```python
from build123d import *

# Parameters (mm, degrees)
BOSS_EXTRUDE2_DEPTH = 50
CUT_EXTRUDE2_DEPTH  = 63
SKETCH6_W           = 25
SKETCH6_H           = 16.790562981
BOSS_EXTRUDE4_DEPTH = 16
CUT_EXTRUDE8_DEPTH  = 25
SKETCH11_W          = 19
SKETCH11_H          = 10.094840621
CUT_EXTRUDE9_DEPTH  = 25


with BuildPart() as part:
    # Sketch1 → Boss-Extrude2 (new body)
    with BuildSketch(Plane(origin=(0, 0, 0), x_dir=(1, 0, 0), z_dir=(0, 1, 0))):
        Polygon((0, 0), (63, 0), (63, 25), (48, 25), (48, 50), (63, 50), (63, 75), (0, 75), align=None)
    extrude(amount=BOSS_EXTRUDE2_DEPTH)

    # Sketch3 → Cut-Extrude2 (cut)
    with BuildSketch(Plane(origin=(63, 0, 0), x_dir=(0, 0, -1), z_dir=(1, 0, 0))):
        Polygon((75, 50), (0, 13.523152522), (0, 50), align=None)
    extrude(amount=-CUT_EXTRUDE2_DEPTH, mode=Mode.SUBTRACT)

    # Sketch6 → Boss-Extrude4 (add)
    with BuildSketch(Plane(origin=(0, 10.936247914, 5.318931295), x_dir=(1, 0, 0), z_dir=(0, 0.8992805495570562, 0.437372259280763))):
        with Locations((31.5, 40.412961178)):
            Rectangle(SKETCH6_W, SKETCH6_H)
    extrude(amount=BOSS_EXTRUDE4_DEPTH)

    # Sketch10 → Cut-Extrude8 (cut)
    with BuildSketch(Plane(origin=(44, 0, 0), x_dir=(0, 0, -1), z_dir=(1, 0, 0))):
        Polygon((38.573371995, 32.283619282), (19.90226542, 32.283619282), (16.475989141, 39.328381609), (31.575415847, 46.672108075), align=None)
    extrude(amount=-CUT_EXTRUDE8_DEPTH, mode=Mode.SUBTRACT)

    # Sketch11 → Cut-Extrude9 (cut)
    with BuildSketch(Plane(origin=(0, 0, -75), x_dir=(-1, 0, 0), z_dir=(0, 0, -1))):
        with Locations((-31.5, 44.952579689)):
            Rectangle(SKETCH11_W, SKETCH11_H)
    extrude(amount=-CUT_EXTRUDE9_DEPTH, mode=Mode.SUBTRACT)


solid = part.part
```
For this review, take the finished solid that the model builds, in its own axes (mm). A direction names the side the tool comes from. Give positions to 0.01 mm unless a question says otherwise; leave off trailing zeros. Write each loop counter-clockwise with the first axis right and the second up, starting at its lowest first coordinate (ties: lowest second). Pieces come first, ordered by that corner, then holes.
Item 1: The part is to be moulded in two halves that separate along Z. For faces 1 (the face through (48, 14, -37)), 2 (the face through (63, 10, -12)), 3 (the face through (31, 7, 0)), 4 (the face through (32, 25, -75)), say which applies: +Z half, -Z half, draft (parallel to the pull), parting line (faces both ways), or undercut.
Item 2: Take a section at D-D (z = -68.5). Give the boundary of the cut face in (x, y), and give its area (3 significant figures).
Item 3: Insertion check: P1, Ø5.5, axis at x = 33.5, z = -31, coming from the +Y side; P2, Ø1.5, axis at x = 36, y = 17, coming from the +Z side; P3, Ø9.5, axis at x = 28.5, z = -62, coming from the +Y side. Each pin has a flat end and moves straight along its axis. Give the tip position at first contact, or say it passes through.
Item 4: Machinability: for faces 5 (the face through (31.325, 28.56, -21.713)), 6 (the face through (44, 31, -28)), 7 (the face through (55, 19, -50)), which of the approach directions +Z, -Z, +X, -X, +Y, -Y give a long, thin tool a straight path to every point of the face, cutting with its end or side? Answer none if there is none.
Item 5: Take a section at B-B (y = 43). Give the boundary of the cut face in (x, z).
Item 6: Wall thickness on probe 1 along X at (y, z) = (24.5, -38.5); probe 2 along Y at (x, z) = (36, -27); probe 3 along Z at (x, y) = (57, 7): over which ranges is each line inside the solid? List them lowest first.
Item 7: Take a section at A-A (x = 49). Give the boundary of the cut face in (y, z).
Item 8: Take a section at C-C (y = 12.5). Give the boundary of the cut face in (x, z), and give its area (3 significant figures).
Established:
1. face 1: undercut
1. face 2: draft
1. face 3: +Z half
1. face 4: -Z half
2. outline: (0, 0) - (63, 0) - (63, 46.84) - (41, 46.84) - (41, 39.91) - (22, 39.91) - (22, 46.84) - (0, 46.84) - close
2. area: 2,820 mm2
3. P1: stops at y = 32.28
3. P2: stops at z = -5.61
3. P3: stops at y = 39.91
4. face 5: +Z, +X, -X
4. face 6: +Z, +X, +Y
4. face 7: +X, +Y, -Y
5. outline: (0, -75) - (22, -75) - (22, -60.61) - (0, -60.61) - close; (41, -75) - (63, -75) - (63, -60.61) - (41, -60.61) - close
6. probe 1: x = 0 to 48
6. probe 2: y = 0 to 32.28
6. probe 3: z = -75 to -50, -25 to 0
7. outline: (0, -75) - (50, -75) - (37.84, -50) - (0, -50) - close; (0, -25) - (25.68, -25) - (13.52, 0) - (0, 0) - close
8. outline: (0, -75) - (63, -75) - (63, -50) - (48, -50) - (48, -25) - (63, -25) - (63, 0) - (0, 0) - close
8. area: 4,350 mm2
